Autodesk Inventor part; units mm, degrees
ref_plane "YZ Plane" through (0, 0, 0) normal (1, 0, 0) x (0, 1, 0)
ref_plane "XZ Plane" through (0, 0, 0) normal (0, 1, 0) x (-1, 0, 0)
ref_plane "XY Plane" through (0, 0, 0) normal (0, 0, 1) x (1, 0, 0)
sketch "スケッチ1" plane through (0, 0, 0) normal (1, 0, 0) x (0, 1, 0)
  line L0 (0, 0) -> (0, 58.5) construction
  line L1 (16.75, 56.5) -> (16.75, -4)
  line L2 (16.75, -4) -> (15.5, -4)
  line L3 (6.1, -4) -> (6.1, -1.4142)
  line L4 (5.714, 0) -> (4.6858, 0) construction
  line L5 (4.6858, 0) -> (-4.6858, 0)
  line L6 (-6.1, 0) -> (-6.1, -1.4142) construction
  line L7 (-6.1, -4) -> (-12.5, -4)
  line L8 (-16.75, -4) -> (-16.75, 56.5)
  arc A0 (-4.6858, 0) -> (-6.1, -1.4142) centre (-5.3929, -0.7071) ccw
  line L9 (14.75, 58.5) -> (5.25, 58.5)
  line L10 (16.75, 56.5) -> (14.75, 58.5)
  line L11 (-16.75, 56.5) -> (-14.75, 58.5)
  line L12 (13.5, 55.25) -> (-13.5, 55.25) construction
  line L13 (-13.5, 55.25) -> (-13.5, 3.25) construction
  line L14 (-13.5, 3.25) -> (13.5, 3.25) construction
  line L15 (13.5, 3.25) -> (13.5, 55.25) construction
  line L16 (0, 29.25) -> (21.0927, 29.25) construction
  line L17 (14, -2) -> (-14, -2) construction
  arc A1 (12.5, -4) -> (15.5, -4) centre (14, -2) ccw
  line L18 (15.5, -4) -> (12.5, -4) construction
  line L19 (12.5, -4) -> (6.1, -4)
  arc A2 (-15.5, -4) -> (-12.5, -4) centre (-14, -2) ccw
  line L20 (-12.5, -4) -> (-15.5, -4) construction
  line L21 (-15.5, -4) -> (-16.75, -4)
  line L22 (6.25, 52.5) -> (-6.25, 52.5)
  line L23 (-11.25, 47.5) -> (-11.25, 12)
  line L24 (-11.25, 12) -> (11.25, 12)
  line L25 (11.25, 12) -> (11.25, 47.5)
  arc A3 (11.25, 47.5) -> (6.25, 52.5) centre (6.25, 47.5) ccw
  arc A4 (-6.25, 52.5) -> (-11.25, 47.5) centre (-6.25, 47.5) ccw
  line L26 (6.1, -1.4142) -> (6.1, -0.7071) construction
  line L27 (-4.6858, 0) -> (-6.1, 0) construction
  line L28 (-6.1, -1.4142) -> (-6.1, -4)
  line L29 (6.1, -1.4142) -> (6.1, 0) construction
  line L30 (6.1, 0) -> (4.6858, 0) construction
  arc A5 (6.1, -1.4142) -> (4.6858, 0) centre (5.3929, -0.7071) ccw
  line L31 (-14.75, 58.5) -> (-14.75, 62.5)
  line L32 (-14.75, 62.5) -> (3.25, 62.5)
  line L33 (3.25, 62.5) -> (3.25, 58.5)
  arc A6 (3.25, 58.5) -> (5.25, 58.5) centre (4.25, 58.5) ccw
  line L34 (3.25, 58.5) -> (-14.75, 58.5) construction
  line L35 (5.25, 58.5) -> (3.25, 58.5) construction
  line L36 (0.75, 60.5) -> (-12.25, 60.5) construction
  point P0 (16.75, 58.5)
  point P1 (-6.0944, 0.0056)
  point P2 (-16.75, 58.5)
  point P3 (-5.75, 60.5)
  dimension "d3" = 12.2
  dimension "d5" = 33.5
  dimension "d6" = 4
  dimension "d7" = 58.5
  dimension "d8" = 2
  dimension "d9" = 2
  dimension "d10" = 2
  dimension "d11" = 2
  dimension "d12" = 27
  dimension "d13" = 52
  dimension "d14" = 2
  dimension "d15" = 28
  dimension "d16" = 2.5
  dimension "d33" = 5
  dimension "d34" = 5.5
  dimension "d35" = 6
  dimension "d36" = 12
  dimension "d37" = 1
  dimension "d60" = 1
  dimension "d61" = 18
  dimension "d62" = 4
  dimension "d63" = 2
  dimension "d64" = 2.5
  dimension "d65" = 2.5
extrude "押し出し1" add sketch "スケッチ1" against normal blind 1.2
sketch "スケッチ2" plane through (-1.2, 0, 0) normal (1, 0, 0) x (0, 0, -1)
  line L0 (-58.5, 14.75) -> (-58.5, -14.75) construction
  line L1 (-56.5, -16.75) -> (4, -16.75) construction
  line L2 (4, 16.75) -> (-56.5, 16.75) construction
  line L3 (0, -4.6858) -> (0, 4.6858) construction
  line L4 (-0.8, 13.9287) -> (-0.8, -13.9287)
  line L5 (-2.8213, -15.95) -> (-55.6787, -15.95)
  line L6 (-57.7, -13.9287) -> (-57.7, 13.9287)
  line L7 (-55.6787, 15.95) -> (-2.8213, 15.95)
  line L8 (-1.2393, -14.9893) -> (-1.7607, -15.5107)
  line L9 (-1.2393, 14.9893) -> (-1.7607, 15.5107)
  line L10 (-56.7393, 15.5107) -> (-57.2607, 14.9893)
  line L11 (-57.2607, -14.9893) -> (-56.7393, -15.5107)
  arc A0 (-1.2393, -14.9893) -> (-0.8, -13.9287) centre (-2.3, -13.9287) ccw
  arc A1 (-2.8213, -15.95) -> (-1.7607, -15.5107) centre (-2.8213, -14.45) ccw
  arc A2 (-56.7393, -15.5107) -> (-55.6787, -15.95) centre (-55.6787, -14.45) ccw
  arc A3 (-57.7, -13.9287) -> (-57.2607, -14.9893) centre (-56.2, -13.9287) ccw
  arc A4 (-55.6787, 15.95) -> (-56.7393, 15.5107) centre (-55.6787, 14.45) ccw
  arc A5 (-57.2607, 14.9893) -> (-57.7, 13.9287) centre (-56.2, 13.9287) ccw
  arc A6 (-1.7607, 15.5107) -> (-2.8213, 15.95) centre (-2.8213, 14.45) ccw
  arc A7 (-0.8, 13.9287) -> (-1.2393, 14.9893) centre (-2.3, 13.9287) ccw
  arc A8 (-52.5, -6.25) -> (-47.5, -11.25) centre (-47.5, -6.25) ccw
  line L12 (-12, -11.25) -> (-47.5, -11.25)
  line L13 (-12, 11.25) -> (-12, -11.25)
  line L14 (-47.5, 11.25) -> (-12, 11.25)
  arc A9 (-47.5, 11.25) -> (-52.5, 6.25) centre (-47.5, 6.25) ccw
  line L15 (-52.5, -6.25) -> (-52.5, 6.25)
  point P0 (0, 0)
  point P1 (-0.8, -14.55)
  point P2 (-2.2, -15.95)
  point P3 (-0.8, -15.95)
  point P4 (-0.8, 14.55)
  point P5 (-2.2, 15.95)
  point P6 (-0.8, 15.95)
  point P7 (-56.3, 15.95)
  point P8 (-57.7, 14.55)
  point P9 (-57.7, 15.95)
  point P10 (-57.7, -14.55)
  point P11 (-56.3, -15.95)
  point P12 (-57.7, -15.95)
  point P13 (52.5, -6.25)
  point P14 (47.5, -11.25)
  point P15 (47.5, 11.25)
  point P16 (52.5, 6.25)
  dimension "d38" = 1.4
  dimension "d39" = 1.4
  dimension "d40" = 1.4
  dimension "d41" = 1.4
  dimension "d42" = 1.4
  dimension "d43" = 1.4
  dimension "d44" = 1.4
  dimension "d45" = 1.4
  dimension "d46" = 1.5
  dimension "d48" = 0.8
  dimension "d50" = 0.8
  dimension "d53" = 0.8
  dimension "d54" = 0.8
extrude "押し出し2" add sketch "スケッチ2" against normal blind 0.8
hole "穴1" at (0, 13.5, 55.25) at (0, -13.5, 55.25) at (0, -13.5, 3.25) at (0, 13.5, 3.25) direction (-1, 0, 0) diameter 2.6 end through all
hole "穴2" at (0, 14, -2) at (0, -14, -2) at (0, -12.25, 60.5) at (0, 0.75, 60.5) direction (-1, 0, 0) diameter 2 end through all
sketch "スケッチ3" plane through (0, 0, 0) normal (1, 0, 0) x (0, 0, -1)
  circle A0 centre (-13.5, 0.8) radius 12.2
  line L0 (4, 16.75) -> (-56.5, 16.75)
  line L1 (0, -4.6858) -> (0, 4.6858)
  point P0 (0, 0)
  dimension "d55" = 24.4
  dimension "d56" = 15.95
  dimension "d57" = 13.5
extrude "押し出し3" cut sketch "スケッチ3" against normal blind 10
hole "穴3" at (0, -5.75, 60.5) direction (-1, 0, 0) diameter 1.5 end through all
sketch "スケッチ4" plane through (-2, 0, 0) normal (-1, 0, 0) x (0, 0, 1)
  line L0 (22.7958, 14.95) -> (49.25, 14.95)
  line L1 (49.25, 14.95) -> (49.25, 12.25) construction
  line L2 (49.25, 12.25) -> (22.7958, 12.25)
  line L3 (22.7958, 12.25) -> (22.7958, 14.95) construction
  line L4 (53.5, 7.5) -> (56.7, 7.5) construction
  line L5 (56.7, 7.5) -> (56.7, -7.5)
  line L6 (56.7, -7.5) -> (53.5, -7.5) construction
  line L7 (53.5, -7.5) -> (53.5, 7.5)
  line L8 (18.4072, -12.25) -> (49.25, -12.25)
  line L9 (49.25, -12.25) -> (49.25, -14.95) construction
  line L10 (49.25, -14.95) -> (18.4072, -14.95)
  line L11 (18.4072, -14.95) -> (18.4072, -12.25) construction
  arc A0 (22.7958, 14.95) -> (22.7958, 12.25) centre (22.7958, 13.6) ccw
  arc A1 (49.25, 12.25) -> (49.25, 14.95) centre (49.25, 13.6) ccw
  arc A2 (56.7, 7.5) -> (53.5, 7.5) centre (55.1, 7.5) ccw
  arc A3 (53.5, -7.5) -> (56.7, -7.5) centre (55.1, -7.5) ccw
  arc A4 (49.25, -14.95) -> (49.25, -12.25) centre (49.25, -13.6) ccw
  arc A5 (18.4072, -12.25) -> (18.4072, -14.95) centre (18.4072, -13.6) ccw
  line L12 (55.6787, 15.95) -> (2.8213, 15.95) construction
  line L13 (19.7958, 11.25) -> (47.5, 11.25) construction
  line L14 (52.5, 6.25) -> (52.5, -6.25) construction
  line L15 (57.7, -13.9287) -> (57.7, 13.9287) construction
  line L16 (47.5, -11.25) -> (15.4072, -11.25) construction
  line L17 (2.8213, -15.95) -> (55.6787, -15.95) construction
  circle A6 centre (55.25, -13.5) radius 1.3 construction
  circle A7 centre (55.25, 13.5) radius 1.3 construction
  point P0 (0, 0)
  dimension "d73" = 1
  dimension "d74" = 1
  dimension "d75" = 1.35
  dimension "d76" = 1
  dimension "d77" = 1
  dimension "d78" = 1.6
  dimension "d79" = 1
  dimension "d80" = 1
  dimension "d81" = 3
  dimension "d82" = 3
  dimension "d83" = 6
  dimension "d84" = 6
  dimension "d85" = 6
  dimension "d86" = 6
extrude "押し出し4" cut sketch "スケッチ4" against normal blind 1.25
chamfer "面取り1" distance 0.2 angle 45 6 edges at (-0.6, 16.75, -4) (-0.6, -16.75, -4) (-0.6, -6.1, -4) (-0.6, 6.1, -4) (-0.6, 3.25, 62.5) (-0.6, -14.75, 62.5)
properties part number "SERVO_BOTTOM_SPACER"
Geometry: final body of the model. Coordinates: model frame, mm. A direction names the side the tool comes from. Give positions to 0.01 mm unless a question says otherwise; leave off trailing zeros. Loops run counter-clockwise (first coordinate to the right, second up) from the corner with the lowest first, then second, coordinate; pieces in that order, holes last. Notation, with made-up numbers: M 71.25,65 L 102.25,65 A13 cw 102.25,87 Z; hole C 88.25,76 d4. An arc over 180 degrees is marked long. Put each result on its own line as item: value. Start each with the question number.
1) Ray query, line 1 along Y through (x, z) = (-0.7, -2); line 2 along Y through (x, z) = (-0.95, 60.5); line 3 along Z through (x, y) = (-1.35, 0.8). Return the intervals inside material, ascending.
2) Access query for faces 4 (the flat face through (-1, 16.75, 27)), 5 (the flat face through (-1, -11.25, 32)), 6 (the cylindrical face through (-1.384, 13.63, 21.446)). Directions: +Z, -Z, +X, -X, +Y, -Y. A direction counts if a zero-diameter tool reaches every point of the face in a straight line with its end or side. Return the directions, or none.
3) Cut plane C-C (y = 10). Output: boundary loops of the cut face in (x, z), then the cut area to 3 significant figures.
4) Contact query for flat-ended pins moving along their axis: pin 1 (17 mm diameter, centred on y = 5, z = 32, fed in from -X); pin 2 (0.6 mm diameter, centred on x = -0.5, z = 60.5, fed in from +Y). Output: stop coordinate, or through.
5) Cut plane B-B (z = 60.5). Output: boundary loops of the cut face in (x, y), then the cut area to 3 significant figures.
6) Pull-direction query (Y, two-part tool) for faces 1 (the flat face through (-1, -14.75, 60)), 2 (the flat face through (-0.59, 15.76, 57.49)), 3 (the cylindrical face through (-0.6, 6.1, 0)); classes: pulls with the +Y half, pulls with the -Y half, needs draft (parallel to the pull), parting line crosses it, or undercut.
7) Cut plane A-A (z = 28). Output: boundary loops of the cut face in (x, y).
8) Cut plane D-D (z = 14.5). Output: boundary loops of the cut face in (x, y).
Verdict:
1. line 1: -16.75 to -15, -13 to -6.1, 6.1 to 13, 15 to 16.75
1. line 2: -14.75 to -13.25, -11.25 to -6.5, -5 to -0.25, 1.75 to 3.25
1. line 3: 0.8 to 1.3, 52.5 to 53.5, 56.7 to 57.7
2. face 4: +Z, -Z, +X, -X, +Y
2. face 5: +X, -X
2. face 6: -X
3. outline: M -2,0.8 L -1.2,0.8 L -1.2,-4 L 0,-4 L 0,5.49 L -2,5.49 Z; M -2,50.81 L 0,50.81 L 0,58.5 L -1.2,58.5 L -1.2,57.7 L -2,57.7 Z
3. area: 29.9 mm2
4. pin 1: x = -2
4. pin 2: y = 3.25
5. outline: M -1.2,-14.75 L 0,-14.75 L 0,-13.25 L -1.2,-13.25 Z; M -1.2,-11.25 L 0,-11.25 L 0,-6.5 L -1.2,-6.5 Z; M -1.2,-5 L 0,-5 L 0,-0.25 L -1.2,-0.25 Z; M -1.2,1.75 L 0,1.75 L 0,3.25 L -1.2,3.25 Z
5. area: 15.0 mm2
6. face 1: pulls with the -Y half
6. face 2: pulls with the +Y half
6. face 3: undercut
7. outline: M -2,-15.95 L -1.2,-15.95 L -1.2,-16.75 L 0,-16.75 L 0,-11.25 L -2,-11.25 L -2,-12.25 L -0.75,-12.25 L -0.75,-14.95 L -2,-14.95 Z; M -2,11.25 L 0,11.25 L 0,16.75 L -1.2,16.75 L -1.2,15.95 L -2,15.95 L -2,14.95 L -0.75,14.95 L -0.75,12.25 L -2,12.25 Z
8. outline: M -2,-15.95 L -1.2,-15.95 L -1.2,-16.75 L 0,-16.75 L 0,-11.36 L -2,-11.36 Z; M -2,12.96 L 0,12.96 L 0,16.75 L -1.2,16.75 L -1.2,15.95 L -2,15.95 Z
